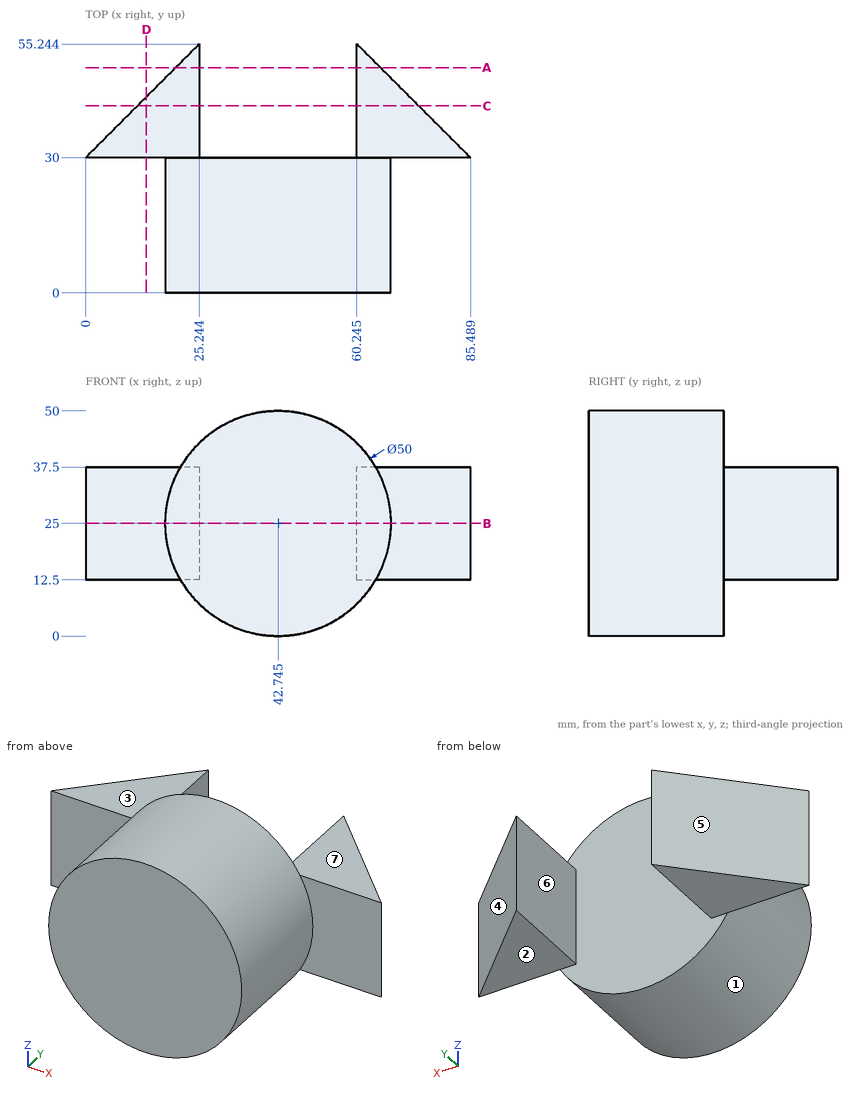
Answer from the drawing. Dimensions are ordinates in mm from the lowest x, y and z of the part. A direction names the side the tool comes from. Round coordinates to 2 decimals unless told otherwise and drop trailing zeros. Loops run counter-clockwise (first coordinate to the right, second up) from the corner with the lowest first, then second, coordinate; pieces in that order, holes last. Notation, with made-up numbers: (60.25, 80) - (111.25, 80) arc R31 ccw to (111.25, 104) - close; hole circle Ø6 at (-1, 68). An arc over 180 degrees is marked (long way). Return JSON: item names as keys, results as strings. Group by question number.
1. The part is cut by section C-C on y = 41.5. Determine the outline of the cut face in (x, z) (1 decimal), then the cut area to 3 significant figures.
2. Which of the six approach directions +Z, -Z, +X, -X, +Y, -Y give full straight-line access (tool end or side, diameter ignored) to the marked faces 1, 2 and 3?
3. Each of these flat-tipped pins is pushed along its axis until it touches: P1, Ø12.5, axis at y = 36.5, z = 19.5, coming from the -X side; P2, Ø8, axis at y = 15.5, z = 43.5, coming from the +X side; P3, Ø12, axis at x = 35, y = 9, coming from the -Z side. Where does it stop, or does it pass through?
4. The mould has two halves that part along X. Classify the marked faces 4, 5, 6 and 7: pulls with the +X half, pulls with the -X half, needs draft (parallel to the pull), parting line crosses it, or undercut.
5. The part is cut by section A-A on y = 50. Determine the outline of the cut face in (x, z) (1 decimal).
6. The part is cut by section D-D on x = 13.5. Determine the outline of the cut face in (y, z).
7. The part is cut by section B-B on z = 25. Determine the outline of the cut face in (x, y) (1 decimal).
8. Consider probe 1 along Y at (x, z) = (58, 30); probe 2 along Z at (x, y) = (66, 33.5); probe 3 along X at (y, z) = (44, 33) (1 decimal). Determine where each line is inside the solid, lowest interval first.
Resolved:
{
 "1": {"outline": "(11.5, 12.5) - (25.2, 12.5) - (25.2, 37.5) - (11.5, 37.5) - close; (60.2, 12.5) - (74, 12.5) - (74, 37.5) - (60.2, 37.5) - close", "area": "687 mm²"},
 "2": {"face 1": "-Y", "face 2": "-Z, +X, -X, +Y", "face 3": "+Z, +X, -X, +Y"},
 "3": {"P1": "stops at x = 0.25", "P2": "stops at x = 63.11", "P3": "stops at z = 0.06"},
 "4": {"face 4": "pulls with the +X half", "face 5": "pulls with the -X half", "face 6": "undercut", "face 7": "needs draft"},
 "5": {"outline": "(20, 12.5) - (25.2, 12.5) - (25.2, 37.5) - (20, 37.5) - close; (60.2, 12.5) - (65.5, 12.5) - (65.5, 37.5) - (60.2, 37.5) - close"},
 "6": {"outline": "(30, 12.5) - (43.5, 12.5) - (43.5, 37.5) - (30, 37.5) - close"},
 "7": {"outline": "(0, 30) - (17.7, 30) - (17.7, 0) - (67.7, 0) - (67.7, 30) - (85.5, 30) - (60.2, 55.2) - (60.2, 30) - (25.2, 30) - (25.2, 55.2) - close"},
 "8": {"probe 1": "y = 0 to 30", "probe 2": "z = 12.5 to 37.5", "probe 3": "x = 14 to 25.2, 60.2 to 71.5"}
}
